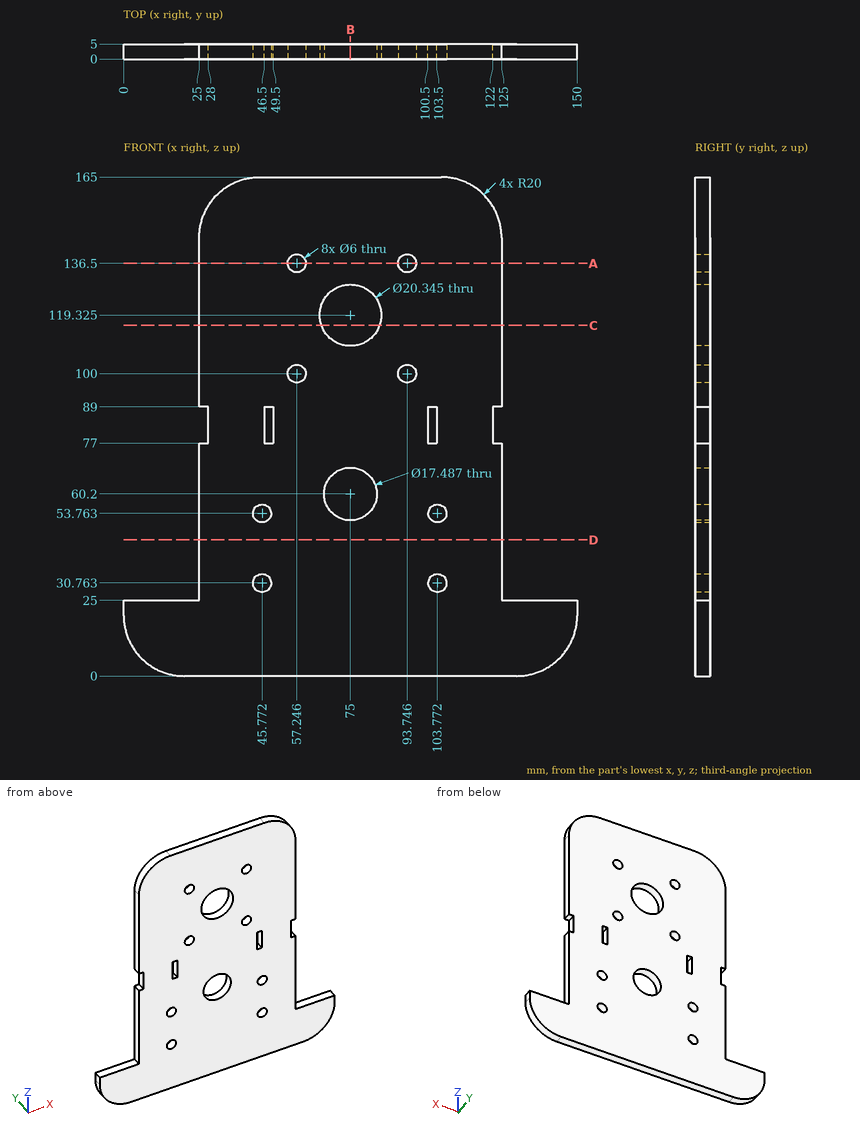
The drawing under review shows one solid part. Ordinate dimensions are in mm from its lowest x, y, z. Round coordinates to 2 decimals unless told otherwise and drop trailing zeros. Order: outer loops, then holes, each group sorted by start corner. A loop starts at its lowest first (then second) coordinate and runs counter-clockwise, first axis right, second up. Notation, with made-up numbers: M -15.75,59.25 L 0.25,59.25 A27 ccw 0.25,77.25 Z; hole C 7,-35 d9. An arc over 180 degrees is marked long. Answer as CSV lines item,"result". Start each with the question number.
1) Add section B-B (x = 75). Give the boundary of the cut face in (y, z), then the cut area to 3 significant figures.
2) For pin 1 Ø2 at (x, y) = (23, 2) entering from +Z; pin 2 Ø7 at (x, z) = (45.77, 30.76) entering from -Y; pin 3 Ø2.5 at (x, y) = (26, 3.5) entering from +Z (1 decimal); pin 4 Ø2.5 at (y, z) = (2, 110.5) entering from +X, all flat-tipped, find the tip position at first contact; note any pin that passes through.
3) Add section A-A (z = 136.5). Give the boundary of the cut face in (x, y).
4) Wall thickness on line 1 along X through (y, z) = (4, 136.5); line 2 along X through (y, z) = (1.9, 31.5); line 3 along X through (y, z) = (0.3, 124.5): over which ranges is each line inside the solid? List them lowest first. Write a range as [from, to].
5) Add section D-D (z = 45). Give the boundary of the cut face in (x, y), then the cut area to 3 significant figures.
6) Add section C-C (z = 116). Give the boundary of the cut face in (x, y).
Resolved:
1,outline,"M 0,0 L 5,0 L 5,51.46 L 0,51.46 Z; M 0,68.94 L 5,68.94 L 5,109.15 L 0,109.15 Z; M 0,129.5 L 5,129.5 L 5,165 L 0,165 Z"
1,area,"636 mm^2"
2,pin 1,"z = 25"
2,pin 2,"y = 0"
2,pin 3,"z = 154.2"
2,pin 4,"x = 125"
3,outline,"M 25,0 L 54.25,0 L 54.25,5 L 25,5 Z; M 60.25,0 L 90.75,0 L 90.75,5 L 60.25,5 Z; M 96.75,0 L 125,0 L 125,5 L 96.75,5 Z"
4,line 1,"[25, 54.25], [60.25, 90.75], [96.75, 125]"
4,line 2,"[25, 42.86], [48.68, 100.86], [106.68, 125]"
4,line 3,"[25, 66.24], [83.76, 125]"
5,outline,"M 25,0 L 125,0 L 125,5 L 25,5 Z"
5,area,"500 mm^2"
6,outline,"M 25,0 L 65.39,0 L 65.39,5 L 25,5 Z; M 84.61,0 L 125,0 L 125,5 L 84.61,5 Z"
